Work out the finished part from the listing and answer in its coordinate system (mm). A direction names the side the tool comes from. Coordinates: 2 decimals unless noted, no trailing zeros. Order: outer loops, then holes, each group sorted by start corner. A loop starts at its lowest first (then second) coordinate and runs counter-clockwise, first axis right, second up. Notation, with made-up numbers: (68.5, -38) - (119.5, -38) arc R36 ccw to (119.5, 0) - close; hole circle Ø5 at (50.5, -7). An arc over 180 degrees is marked (long way). Answer as a JSON object with one key per item and string values. Group by question number.
1) Section C-C (x = 10) is taken. Give the vertices of the cut face in (y, z), plus the area to 3 significant figures.
2) Each of these flat-tipped pins is pushed along its axis until it touches: P1, Ø1.1, axis at x = 5.5, z = 0, coming from the +Y side; P2, Ø4, axis at x = 15.5, y = 0.5, coming from the -Z side; P3, Ø3.5, axis at x = -4.5, z = -0.5, coming from the -Y side. Where does it stop, or does it pass through?
3) A tool of negligible diameter and unlimited length cuts with its end or side. For faces 1 (the face through (-0.9, 3.6, -0.68)), 2 (the face through (23, -3, 0.75)), 3 (the face through (25.4, -1.7, 2.22)), 4 (the face through (23.25, 3, 8)), from which of +Z, -Z, +X, -X, +Y, -Y can it reach the whole face along a straight path? Write none if from no direction.
4) Section D-D (x = 5.19) is taken. Give the vertices of the cut face in (y, z), plus the area to 3 significant figures.
5) The mould has two halves that part along Y. Classify faces 5 (the face through (21, 3.35, -8)), 6 (the face through (-2.575, 5, 0)), 7 (the face through (21, 3, 8.15)): released by +Y, released by -Y, zero draft, split by the parting line, or undercut.
6) Section A-A (y = 9) is taken. Give the vertices of the cut face in (x, z).
7) Section B-B (x = -2) is taken. Give the vertices of the cut face in (y, z).
8) Find the intervals of material crossed by line 1 along X through (y, z) = (7.8, 0); line 2 along X through (y, z) = (5.8, 0) (3 decimals); line 3 along Z through (x, y) = (-4.56, 5.9) (3 decimals), in increasing order.
from build123d import *

# Parameters (mm, degrees)
SKETCH1_W            = 26
SKETCH1_H            = 13.9
BOSS_EXTRUDE1_DEPTH  = 9.8
BOSS_EXTRUDE2_DEPTH  = 4.3
SKETCH4_R            = 4.2
BOSS_EXTRUDE3_DEPTH  = 1
SKETCH5_R            = 3.19
BOSS_EXTRUDE4_DEPTH  = 0.5
SKETCH6_R            = 1.15
BOSS_EXTRUDE5_DEPTH  = 5.4
SKETCH7_R            = 0.49
BOSS_EXTRUDE6_DEPTH  = 5.6
BOSS_EXTRUDE7_DEPTH  = 8.7
BOSS_EXTRUDE8_DEPTH  = 11.5
BOSS_EXTRUDE9_DEPTH  = 3.35
CUT_EXTRUDE1_DEPTH   = 35.297084424
BOSS_EXTRUDE10_START = -2.3
BOSS_EXTRUDE10_DEPTH = 1
BOSS_EXTRUDE11_DEPTH = 2.85
SKETCH15_R           = 0.65
CUT_EXTRUDE2_DEPTH   = 41.713695484
SKETCH14_R           = 1.665
SKETCH14_R_2         = 0.65
BOSS_EXTRUDE12_DEPTH = 1.8
BOSS_EXTRUDE13_DEPTH = 0.68
BOSS_EXTRUDE14_DEPTH = 0.5
SKETCH18_R           = 1.2
BOSS_EXTRUDE15_DEPTH = 0.35
SKETCH20_W           = 4.77
SKETCH20_H           = 1.47
BOSS_EXTRUDE16_DEPTH = 8.15
SKETCH21_R           = 1.4
BOSS_EXTRUDE17_DEPTH = 1
BOSS_EXTRUDE18_START = -1
SKETCH22_R           = 1.4
BOSS_EXTRUDE18_DEPTH = 1.5


with BuildPart() as part:
    # Sketch1 → Boss-Extrude1 (new body)
    with BuildSketch(Plane(origin=(0, 0, 0), x_dir=(1, 0, 0), z_dir=(0, 1, 0))):
        with Locations((13, 0)):
            Rectangle(SKETCH1_W, SKETCH1_H)
    extrude(amount=BOSS_EXTRUDE1_DEPTH)

    # Sketch2 → Boss-Extrude2 (add)
    with BuildSketch(Plane(origin=(0, 9.8, 0), x_dir=(1, 0, 0), z_dir=(0, 1, 0))):
        with BuildLine():
            Line((26, -6.95), (26, 6.95))
            Line((26, 6.95), (12.1, 6.95))
            Line((12.1, 6.95), (12.1, 5.1))
            ThreePointArc((12.1, 5.1), (7.9, 0), (12.1, -5.1))
            Line((12.1, -5.1), (12.1, -6.95))
            Line((12.1, -6.95), (26, -6.95))
        make_face()
    extrude(amount=BOSS_EXTRUDE2_DEPTH)

    # Sketch4 → Boss-Extrude3 (add)
    with BuildSketch(Plane(origin=(0, 14.1, 0), x_dir=(1, 0, 0), z_dir=(0, 1, 0))):
        with Locations(Location((19.6, 0, 0), (0, 0, 270))):
            Circle(SKETCH4_R)
    extrude(amount=BOSS_EXTRUDE3_DEPTH)

    # Sketch5 → Boss-Extrude4 (add)
    with BuildSketch(Plane(origin=(0, 15.1, 0), x_dir=(1, 0, 0), z_dir=(0, 1, 0))):
        with Locations(Location((19.6, 0, 0), (0, 0, 270))):
            Circle(SKETCH5_R)
    extrude(amount=BOSS_EXTRUDE4_DEPTH)

    # Sketch6 → Boss-Extrude5 (add)
    with BuildSketch(Plane(origin=(0, 15.6, 0), x_dir=(1, 0, 0), z_dir=(0, 1, 0))):
        Polygon((18.680674442, 2.829393136), (19.230241972, 2.334560309), (19.6, 2.975), (19.969758028, 2.334560309), (20.519325558, 2.829393136), (20.673079592, 2.10603728), (21.348661126, 2.406825558), (21.271360649, 1.671360649), (22.006825558, 1.748661126), (21.70603728, 1.073079592), (22.429393136, 0.919325558), (21.934560309, 0.369758028), (22.575, 0), (21.934560309, -0.369758028), (22.429393136, -0.919325558), (21.70603728, -1.073079592), (22.006825558, -1.748661126), (21.271360649, -1.671360649), (21.348661126, -2.406825558), (20.673079592, -2.10603728), (20.519325558, -2.829393136), (19.969758028, -2.334560309), (19.6, -2.975), (19.230241972, -2.334560309), (18.680674442, -2.829393136), (18.526920408, -2.10603728), (17.851338874, -2.406825558), (17.928639351, -1.671360649), (17.193174442, -1.748661126), (17.49396272, -1.073079592), (16.770606864, -0.919325558), (17.265439691, -0.369758028), (16.625, 0), (17.265439691, 0.369758028), (16.770606864, 0.919325558), (17.49396272, 1.073079592), (17.193174442, 1.748661126), (17.928639351, 1.671360649), (17.851338874, 2.406825558), (18.526920408, 2.10603728), align=None)
        with Locations(Location((19.6, 0, 0), (0, 0, 90))):
            Circle(SKETCH6_R, mode=Mode.SUBTRACT)
    extrude(amount=BOSS_EXTRUDE5_DEPTH)

    # Sketch7 → Boss-Extrude6 (add)
    with BuildSketch(Plane(origin=(0, 9.8, 0), x_dir=(1, 0, 0), z_dir=(0, 1, 0))):
        with Locations(Location((5.19, 0, 0), (0, 0, 90))):
            Circle(SKETCH7_R)
    extrude(amount=BOSS_EXTRUDE6_DEPTH)

    # Sketch8 → Boss-Extrude7 (add)
    with BuildSketch(Plane.XZ):
        with BuildLine():
            Line((11.5, 3.725), (11.5, -3.725))
            ThreePointArc((11.5, -3.725), (9.018155549, -6.089531686), (5.7, -6.95))
            Line((5.7, -6.95), (0, -6.95))
            Line((0, -6.95), (0, 6.95))
            Line((0, 6.95), (5.7, 6.95))
            ThreePointArc((5.7, 6.95), (9.018155549, 6.089531686), (11.5, 3.725))
        make_face()
    extrude(amount=BOSS_EXTRUDE7_DEPTH)

    # Sketch9 → Boss-Extrude8 (add)
    with BuildSketch(Plane.XZ.offset(8.7)):
        with BuildLine():
            Line((0.5, 3.382306905), (0.5, -3.382306905))
            ThreePointArc((0.5, -3.382306905), (5.48, -6.02), (10.46, -3.382306905))
            Line((10.46, -3.382306905), (10.46, 3.382306905))
            ThreePointArc((10.46, 3.382306905), (5.48, 6.02), (0.5, 3.382306905))
        make_face()
    extrude(amount=BOSS_EXTRUDE8_DEPTH)

    # Sketch10 → Boss-Extrude9 (add)
    with BuildSketch(Plane.XZ):
        Polygon((26, 2.22), (26, -2.22), (24.91, -2.22), (24.91, -0.75), (21.49, -0.75), (21.49, -2.22), (20.4, -2.22), (20.4, 2.22), (21.49, 2.22), (21.49, 0.75), (24.91, 0.75), (24.91, 2.22), align=None)
    extrude(amount=BOSS_EXTRUDE9_DEPTH)

    # Sketch11 → Cut-Extrude1 (cut, through all)
    with BuildSketch(Plane(origin=(0, 0, -0.75), x_dir=(-1, 0, 0), z_dir=(0, 0, -1))):
        with BuildLine():
            Line((-24.2, 0), (-24.2, -1.85))
            ThreePointArc((-24.2, -1.85), (-23.2, -2.85), (-22.2, -1.85))
            Line((-22.2, -1.85), (-22.2, 0))
            Line((-22.2, 0), (-24.2, 0))
        make_face()
    extrude(amount=-CUT_EXTRUDE1_DEPTH, mode=Mode.SUBTRACT)

    # Sketch12 → Boss-Extrude10 (add)
    with BuildSketch(Plane(origin=(0, 9.8, 0), x_dir=(1, 0, 0), z_dir=(0, 1, 0)).offset(BOSS_EXTRUDE10_START)):
        with BuildLine():
            Line((0, 6.876790543), (0, -6.876790543))
            ThreePointArc((0, -6.876790543), (-6.7, 0), (0, 6.876790543))
        make_face()
    extrude(amount=-BOSS_EXTRUDE10_DEPTH)

    # Sketch13 → Boss-Extrude11 (add)
    with BuildSketch(Plane(origin=(0, 7.5, 0), x_dir=(1, 0, 0), z_dir=(0, 1, 0))):
        with BuildLine():
            Line((-6.05, 0.917823512), (-6.05, -0.917823512))
            ThreePointArc((-6.05, -0.917823512), (-2.81, 0), (-6.05, 0.917823512))
        make_face()
    extrude(amount=BOSS_EXTRUDE11_DEPTH)

    # Sketch15 → Cut-Extrude2 (cut, through all)
    with BuildSketch(Plane(origin=(0, 10.35, 0), x_dir=(1, 0, 0), z_dir=(0, 1, 0))):
        with Locations(Location((-4.56, 0, 0), (0, 0, 270))):
            Circle(SKETCH15_R)
    extrude(amount=-CUT_EXTRUDE2_DEPTH, mode=Mode.SUBTRACT)

    # Sketch14 → Boss-Extrude12 (add)
    with BuildSketch(Plane.XZ.offset(-6.5)):
        with Locations(Location((-4.56, 0, 0), (0, 0, 90))):
            Circle(SKETCH14_R)
        with Locations(Location((-4.56, 0, 0), (0, 0, 90))):
            Circle(SKETCH14_R_2, mode=Mode.SUBTRACT)
    extrude(amount=BOSS_EXTRUDE12_DEPTH)

    # Sketch16 → Boss-Extrude13 (add, symmetric)
    with BuildSketch(Plane.XY):
        with BuildLine():
            Line((-3.2, 6.5), (-3.2, 4.7))
            ThreePointArc((-3.2, 4.7), (-2.636457892, 3.039858484), (-1.178739757, 2.065842366))
            Line((-1.178739757, 2.065842366), (0, 1.75))
            Line((0, 1.75), (0, 6.5))
            Line((0, 6.5), (-0.625, 6.5))
            Line((-0.625, 6.5), (-0.625, 4.5))
            ThreePointArc((-0.625, 4.5), (-1.6, 3.525), (-2.575, 4.5))
            Line((-2.575, 4.5), (-2.575, 6.5))
            Line((-2.575, 6.5), (-3.2, 6.5))
        make_face()
    extrude(amount=BOSS_EXTRUDE13_DEPTH, both=True)

    # Sketch17 → Boss-Extrude14 (add, symmetric)
    with BuildSketch(Plane.XY):
        Polygon((11.5, -8.7), (15.9, -1), (20.4, -1), (20.4, 0), (11.5, 0), align=None)
    extrude(amount=BOSS_EXTRUDE14_DEPTH, both=True)

    # Sketch18 → Boss-Extrude15 (add)
    with BuildSketch(Plane(origin=(0, 14.1, 0), x_dir=(1, 0, 0), z_dir=(0, 1, 0))):
        with Locations(Location((13.096428571, 0, 0), (0, 0, 270))):
            Circle(SKETCH18_R)
    extrude(amount=BOSS_EXTRUDE15_DEPTH)

    # Sketch20 → Boss-Extrude16 (add, symmetric)
    with BuildSketch(Plane.XY):
        with Locations((4.945, 2.615)):
            Rectangle(SKETCH20_W, SKETCH20_H)
        with Locations((20.865, 2.615)):
            Rectangle(SKETCH20_W, SKETCH20_H)
    extrude(amount=BOSS_EXTRUDE16_DEPTH, both=True)

    # Sketch21 → Boss-Extrude17 (add)
    with BuildSketch(Plane.XZ):
        with Locations((19.7, 0)):
            Circle(SKETCH21_R)
    extrude(amount=BOSS_EXTRUDE17_DEPTH)

    # Sketch22 → Boss-Extrude18 (add)
    with BuildSketch(Plane.XZ.offset(1).offset(BOSS_EXTRUDE18_START)):
        with Locations((12, 0)):
            Circle(SKETCH22_R)
    extrude(amount=BOSS_EXTRUDE18_DEPTH)


solid = part.part
Report:
{
 "1": {"outline": "(-20.2, -3.98) - (-8.7, -3.98) - (-8.7, -5.43) - (0, -5.43) - (0, -6.95) - (9.8, -6.95) - (9.8, -4.17) - (14.1, -4.17) - (14.1, 4.17) - (9.8, 4.17) - (9.8, 6.95) - (0, 6.95) - (0, 5.43) - (-8.7, 5.43) - (-8.7, 3.98) - (-20.2, 3.98) - close", "area": "358 mm²"},
 "2": {"P1": "stops at y = 15.4", "P2": "stops at z = -6.95", "P3": "stops at y = 3.2"},
 "3": {"face 1": "-Z, -Y", "face 2": "+Z, -Y", "face 3": "+Z, +X, -Y", "face 4": "+Z, +X, +Y, -Y"},
 "4": {"outline": "(-20.2, -6.01) - (-8.7, -6.01) - (-8.7, -6.95) - (1.88, -6.95) - (1.88, -8.15) - (3.35, -8.15) - (3.35, -6.95) - (9.8, -6.95) - (9.8, -0.49) - (15.4, -0.49) - (15.4, 0.49) - (9.8, 0.49) - (9.8, 6.95) - (3.35, 6.95) - (3.35, 8.15) - (1.88, 8.15) - (1.88, 6.95) - (-8.7, 6.95) - (-8.7, 6.01) - (-20.2, 6.01) - close", "area": "404 mm²"},
 "5": {"face 5": "released by +Y", "face 6": "undercut", "face 7": "zero draft"},
 "6": {"outline": "(-6.05, -0.92) arc R1.75 ccw (long way) to (-6.05, 0.92) - close; (0, -6.95) - (26, -6.95) - (26, 6.95) - (0, 6.95) - close; hole circle Ø1.3 at (-4.56, 0)"},
 "7": {"outline": "(2.44, -0.68) - (3.61, -0.68) - (3.61, 0.68) - (2.44, 0.68) - close; (6.5, -6.52) - (7.5, -6.52) - (7.5, 6.52) - (6.5, 6.52) - close"},
 "8": {"line 1": "x = -6.05 to -5.21, -3.91 to -2.81, 0 to 26", "line 2": "x = -6.225 to -5.21, -3.91 to -2.575, -0.625 to 26", "line 3": "z = -1.665 to -0.65, 0.65 to 1.665"}
}
